CAD build for the part. Positions are in the model's coordinates, mm. Face numbers are marked on the shaded views. A direction names the side the tool comes from. Round coordinates to 2 decimals unless told otherwise and drop trailing zeros. Order: outer loops, then holes, each group sorted by start corner. A loop starts at its lowest first (then second) coordinate and runs counter-clockwise, first axis right, second up.
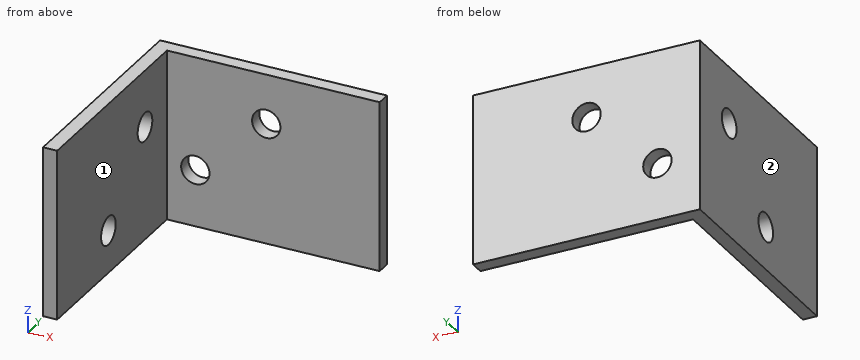
Autodesk Inventor part; units mm, degrees
ref_plane "YZ Plane" through (0, 0, 0) normal (1, 0, 0) x (0, 1, 0)
ref_plane "XZ Plane" through (0, 0, 0) normal (0, 1, 0) x (-1, 0, 0)
ref_plane "XY Plane" through (0, 0, 0) normal (0, 0, 1) x (1, 0, 0)
sketch "Sketch1" plane through (0, 0, 0) normal (0, 0, 1) x (1, 0, 0)
  line L0 (0, 0) -> (50.8, 0)
  line L1 (50.8, 0) -> (50.8, -3.175)
  line L2 (50.8, -3.175) -> (3.175, -3.175)
  line L3 (3.175, -3.175) -> (3.175, -50.8)
  line L4 (3.175, -50.8) -> (0, -50.8)
  line L5 (0, -50.8) -> (0, 0)
  dimension "d0" = 3.175
  dimension "d1" = 3.175
  dimension "d2" = 50.8
  dimension "d3" = 50.8
extrude "Extrusion1" add sketch "Sketch1" along normal blind 38.1
sketch "Sketch2" plane through (0, -50.8, 0) normal (-1, 0, 0) x (0, 0, 1)
  circle A0 centre (25.4, 38.1) radius 3.175
  circle A1 centre (9.525, 22.225) radius 3.175
  line L0 (0, 0) -> (0, 50.8)
  line L1 (0, 50.8) -> (38.1, 50.8)
  line L2 (0, 0) -> (38.1, 0)
  dimension "d6" = 6.35
  dimension "d7" = 6.35
  dimension "d8" = 9.525
  dimension "d9" = 25.4
  dimension "d12" = 12.7
  dimension "d13" = 22.225
extrude "Extrusion2" cut sketch "Sketch2" against normal blind 3.175
sketch "Sketch3" plane through (0, 0, 0) normal (0, 1, 0) x (1, 0, 0)
  circle A0 centre (25.4, -26.9875) radius 3.175
  circle A1 centre (9.525, -12.7) radius 3.175
  line L0 (0, 0) -> (0, -38.1)
  line L1 (50.8, -38.1) -> (0, -38.1)
  line L2 (50.8, 0) -> (50.8, -38.1)
  line L3 (0, 0) -> (50.8, 0)
  dimension "d14" = 9.525
  dimension "d15" = 11.1125
  dimension "d16" = 25.4
  dimension "d17" = 6.35
  dimension "d18" = 6.35
  dimension "d19" = 12.7
extrude "Extrusion3" cut sketch "Sketch3" against normal blind 25.4 contours A0 | A1
properties part number "15102898-16-P-0804" material "Aluminum 6061"
1. Cut at A-A, the plane y = -12.7. Write the cut outline in (x, z) (3 decimals).
2. Drill centre lines: line 1 (Z direction, x = 25.4, y = -2.5); line 2 (X direction, y = -1.65, z = 12.7); line 3 (X direction, y = -21, z = 36) (3 decimals). Where is each one in solid material? Low to high.
3. Pin check, flat tips, straight feed: P1, Ø4, axis at y = -7, z = 33.5, coming from the +X side (3 decimals); P2, Ø10, axis at x = 9.525, z = 12.7, coming from the -Y side (3 decimals). Stop position of each tip, or through.
4. Tool access for the marked faces 1 and 2: list every direction of +Z, -Z, +X, -X, +Y, -Y with a clear straight run to the whole face (end or side of a thin tool).
5. Cut at C-C, the plane x = 25.4. Write the cut outline in (y, z) (1 decimal).
6. Cut at B-B, the plane z = 8.5. Write the cut outline in (x, y) (3 decimals).
7. Cut at D-D, the plane z = 25.4. Write the cut outline in (x, y) (3 decimals).
Outcome:
1. outline: (0, 0) - (3.175, 0) - (3.175, 22.225) - (0, 22.225) - close; (0, 28.575) - (3.175, 28.575) - (3.175, 38.1) - (0, 38.1) - close
2. line 1: z = 0 to 23.81, 30.16 to 38.1
2. line 2: x = 0 to 6.35, 12.7 to 50.8
2. line 3: x = 0 to 3.175
3. P1: stops at x = 3.175
3. P2: stops at y = -3.175
4. face 1: +Z, -Z, +X, -Y
4. face 2: +Z, -Z, -X, +Y, -Y
5. outline: (-3.2, 0) - (0, 0) - (0, 23.8) - (-3.2, 23.8) - close; (-3.2, 30.2) - (0, 30.2) - (0, 38.1) - (-3.2, 38.1) - close
6. outline: (0, -50.8) - (3.175, -50.8) - (3.175, -31.58) - (0, -31.58) - close; (0, -25.57) - (3.175, -25.57) - (3.175, -3.175) - (50.8, -3.175) - (50.8, 0) - (0, 0) - close
7. outline: (0, -50.8) - (3.175, -50.8) - (3.175, -15.875) - (0, -15.875) - close; (0, -9.525) - (3.175, -9.525) - (3.175, -3.175) - (22.65, -3.175) - (22.65, 0) - (0, 0) - close; (28.15, -3.175) - (50.8, -3.175) - (50.8, 0) - (28.15, 0) - close
